Part model, mm, in its own coordinate system. Give positions to 0.01 mm unless a question says otherwise; leave off trailing zeros. Loops run counter-clockwise (first coordinate to the right, second up) from the corner with the lowest first, then second, coordinate; pieces in that order, holes last. Notation, with made-up numbers: (50.25, -5) -> (105.25, -5) arc R22 cw to (105.25, 17) -> close; hole circle Ø3 at (4.25, 37). An arc over 180 degrees is marked (long way). Write item = value, one per line.
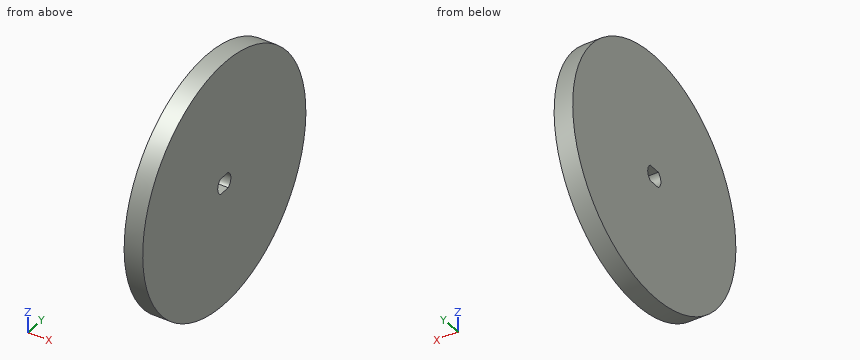
from build123d import *

# Parameters (mm, degrees)
SKETCH1_R  = 18
BASE_DEPTH = 2.7


with BuildPart() as part:
    # Sketch1 → Base (new body)
    with BuildSketch(Plane(origin=(0, 0, 0), x_dir=(0, 0, -1), z_dir=(1, 0, 0))):
        with Locations(Location((0, 0, 0), (0, 0, 180))):
            Circle(SKETCH1_R)
        with BuildLine():
            Line((1.15, 0.883176087), (1.15, -0.883176087))
            ThreePointArc((1.15, -0.883176087), (0, -1.45), (-1.15, -0.883176087))
            Line((-1.15, -0.883176087), (-1.15, 0.883176087))
            ThreePointArc((-1.15, 0.883176087), (0, 1.45), (1.15, 0.883176087))
        make_face(mode=Mode.SUBTRACT)
    extrude(amount=BASE_DEPTH)


solid = part.part
1) Slice it at B-B, the plane z = 0. List the corners of the cut face in (x, y).
Resolved:
outline = (0, -18) -> (2.7, -18) -> (2.7, -1.45) -> (0, -1.45) -> close; (0, 1.45) -> (2.7, 1.45) -> (2.7, 18) -> (0, 18) -> close
2) Drop a flat-ended pin along its axis: P1, Ø0.5, axis at x = 2, y = -0.5, coming from the -Z side. Give the stop position or say it passes through.
Resolved:
P1 = -18
3) Drill centre lines: line 1 along Y through (x, z) = (0.2, -1); line 2 along Z through (x, y) = (1.05, 11); line 3 along Z through (x, y) = (0.6, 1.5). Where is each one in solid material? Low to high. Write a range as [from, to].
Resolved:
line_1 = [-17.97, -1.05], [1.05, 17.97]
line_2 = [-14.25, 14.25]
line_3 = [-17.94, 17.94]
4) Slice it at A-A, the plane y = 0. List the corners of the cut face in (x, z).
Resolved:
outline = (0, -18) -> (2.7, -18) -> (2.7, -1.15) -> (0, -1.15) -> close; (0, 1.15) -> (2.7, 1.15) -> (2.7, 18) -> (0, 18) -> close
5) Slice it at D-D, the plane z = -13. List the corners of the cut face in (x, y), and give its area (3 significant figures).
Resolved:
outline = (0, -12.45) -> (2.7, -12.45) -> (2.7, 12.45) -> (0, 12.45) -> close
area = 67.2 mm²
6) Slice it at C-C, the plane x = 1.6. List the corners of the cut face in (y, z), and give its area (3 significant figures).
Resolved:
outline = circle Ø36 at (0, 0); hole (-0.88, -1.15) -> (0.88, -1.15) arc R1.45 ccw to (0.88, 1.15) -> (-0.88, 1.15) arc R1.45 ccw to start
area = 1,010 mm²
